Verification items for the finished model (mm, model axes). Face numbers are marked on the shaded views. A direction names the side the tool comes from. Coordinates: 2 decimals unless noted, no trailing zeros. Order: outer loops, then holes, each group sorted by start corner. A loop starts at its lowest first (then second) coordinate and runs counter-clockwise, first axis right, second up. Notation, with made-up numbers: (14, 60) -> (22, 60) arc R24 ccw to (22, 84) -> close; hole circle Ø8 at (45, 4). An arc over 180 degrees is marked (long way). Write item = value, one per line. Start each with the question number.
1. Cross-section at D-D on z = 26. Record the cut outline in (x, y), plus the area to 3 significant figures.
2. Cross-section at B-B on x = 48. Record the cut outline in (y, z).
3. Set-up check for the marked faces 1, 2, 3 and 4: record each of +Z, -Z, +X, -X, +Y, -Y from which the full face is reachable in a straight line by a thin tool's end or side.
4. Go/stop test with flat-tipped pins: P1, Ø14.5, axis at x = 32.5, y = 7, coming from the -Z side; P2, Ø2, axis at y = -3.5, z = 17.5, coming from the -X side; P3, Ø1.6, axis at y = 7, z = 19, coming from the +X side; P4, Ø2.5, axis at y = -7.5, z = -1.5, coming from the -X side. Record where each tip stops, or that it passes through.
5. Cross-section at C-C on y = 11.75. Record the cut outline in (x, z).
6. Cross-section at A-A on y = 7. Record the cut outline in (x, z).
7. Thickness scan on line 1 along Z through (x, y) = (59, 10); line 2 along Z through (x, y) = (11, -3.75); line 3 along Z through (x, y) = (45.5, -3). Record the ranges inside material, lowest first. Write a range as from..to.
8. Release check for a two-part mould opening along Z. For the marked faces 5, 6 and 7 record: +Z half, -Z half, draft (parallel to the pull), parting line (faces both ways), or undercut.
from build123d import *

# Parameters (mm, degrees)
BOSS_EXTRUDE1_DEPTH     = 94.99986
SKETCH2_W               = 23
SKETCH2_H               = 14
CUT_EXTRUDE1_DEPTH      = 2
CUT_EXTRUDE2_DEPTH      = 86.037208991
CUT_EXTRUDE2_DEPTH_BACK = 86.037208991
SKETCH4_W               = 25
SKETCH4_H               = 32.499936
SKETCH4_W_2             = 24.99986
SKETCH4_H_2             = 36
SKETCH5_W               = 25
SKETCH5_H               = 2.6
BOSS_EXTRUDE3_DEPTH     = 2
SKETCH6_W               = 24.99986
SKETCH6_H               = 2.5
BOSS_EXTRUDE4_DEPTH     = 2
SKETCH7_R               = 1.5
CUT_EXTRUDE3_DEPTH      = 10
SKETCH8_R               = 1.5
CUT_EXTRUDE4_DEPTH      = 10


with BuildPart() as part:
    # Sketch1 → Boss-Extrude1 (new body)
    with BuildSketch(Plane.ZY.offset(29.759563114)):
        Polygon((-16.355611523, -2.282836071), (-18.355611523, -2.282836071), (-18.355611523, -4.782836071), (18.644388477, -4.782836071), (18.644388477, -2.282836071), (16.644388477, -2.282836071), (16.644388477, 15.217163929), (19.644388477, 15.217163929), (19.644388477, 8.217163929), (17.644388477, 8.217163929), (17.644388477, 5.617163929), (50.644324477, 5.617163929), (50.644324477, 8.217163929), (48.644324477, 8.217163929), (48.644324477, 15.217163929), (52.144324477, 15.217163929), (52.144324477, -13.782836071), (-19.355611523, -13.782836071), (-19.355611523, -0.782836071), (-16.355611523, -0.782836071), align=None)
    extrude(amount=-BOSS_EXTRUDE1_DEPTH)

    # Sketch2 → Cut-Extrude1 (cut)
    with BuildSketch(Plane(origin=(0, 5.617163929, 0), x_dir=(1, 0, 0), z_dir=(0, 1, 0))):
        with Locations((53.740296886, -27.644388477)):
            Rectangle(SKETCH2_W, SKETCH2_H)
    extrude(amount=-CUT_EXTRUDE1_DEPTH, mode=Mode.SUBTRACT)

    # Sketch4 → Cut-Extrude2 (cut, two sides: drawn at the far end of the back side and taken through both)
    with BuildSketch(Plane(origin=(0, -0.782836071, 0), x_dir=(1, 0, 0), z_dir=(0, 1, 0)).offset(-CUT_EXTRUDE2_DEPTH_BACK)):
        with Locations((-17.259563114, -35.894356477)):
            Rectangle(SKETCH4_W, SKETCH4_H)
        with Locations((52.740366886, 1.355611523)):
            Rectangle(SKETCH4_W_2, SKETCH4_H_2)
    extrude(amount=CUT_EXTRUDE2_DEPTH + CUT_EXTRUDE2_DEPTH_BACK, mode=Mode.SUBTRACT)

    # Sketch5 → Boss-Extrude3 (add)
    with BuildSketch(Plane.XY.offset(19.644388477)):
        with Locations((-17.259563114, 6.917163929)):
            Rectangle(SKETCH5_W, SKETCH5_H)
    extrude(amount=-BOSS_EXTRUDE3_DEPTH)

    # Sketch6 → Boss-Extrude4 (add)
    with BuildSketch(Plane(origin=(0, 0, 16.644388477), x_dir=(-1, 0, 0), z_dir=(0, 0, -1))):
        with Locations((-52.740366886, -3.532836071)):
            Rectangle(SKETCH6_W, SKETCH6_H)
    extrude(amount=-BOSS_EXTRUDE4_DEPTH)

    # Sketch7 → Cut-Extrude3 (cut)
    with BuildSketch(Plane(origin=(65.240296886, 0, 0), x_dir=(0, 0, -1), z_dir=(1, 0, 0))):
        with Locations((-40.144324477, 3.217163929)):
            Circle(SKETCH7_R)
    extrude(amount=-CUT_EXTRUDE3_DEPTH, mode=Mode.SUBTRACT)

    # Sketch8 → Cut-Extrude4 (cut)
    with BuildSketch(Plane.ZY.offset(29.759563114)):
        with Locations((-1.355611523, -7.182836071)):
            Circle(SKETCH8_R)
    extrude(amount=-CUT_EXTRUDE4_DEPTH, mode=Mode.SUBTRACT)


solid = part.part
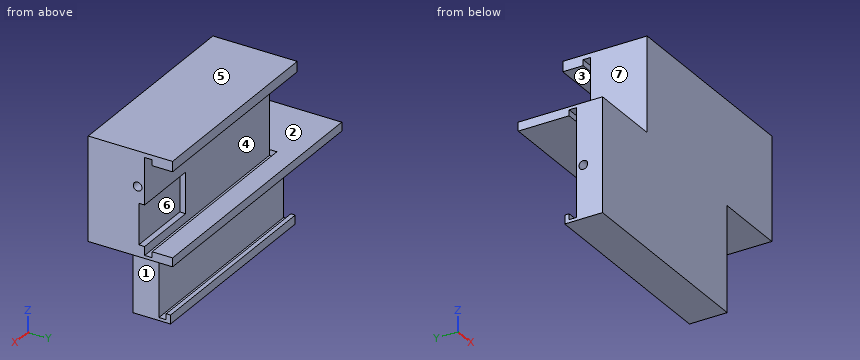
Worked out:
q1.outline = (-4.76, -13.78) -> (65.24, -13.78) -> (65.24, 3.62) -> (42.24, 3.62) -> (42.24, 5.62) -> (-4.76, 5.62) -> close
q1.area = 1,310 mm²
q2.outline = (-13.78, 16.64) -> (15.22, 16.64) -> (15.22, 19.64) -> (8.22, 19.64) -> (8.22, 17.64) -> (5.62, 17.64) -> (5.62, 20.64) -> (3.62, 20.64) -> (3.62, 34.64) -> (5.62, 34.64) -> (5.62, 50.64) -> (8.22, 50.64) -> (8.22, 48.64) -> (15.22, 48.64) -> (15.22, 52.14) -> (-13.78, 52.14) -> close
q3.face_1 = -Z, +X, +Y, -Y
q3.face_2 = -X, +Y
q3.face_3 = +X, -X, +Y
q3.face_4 = +X
q4.P1 = 16.64
q4.P2 = 40.24
q4.P3 = -4.76
q4.P4 = -29.76
q5.outline = (-29.76, 16.64) -> (65.24, 16.64) -> (65.24, 19.64) -> (-29.76, 19.64) -> close; (-4.76, 48.64) -> (65.24, 48.64) -> (65.24, 52.14) -> (-4.76, 52.14) -> close
q6.outline = (-29.76, 16.64) -> (65.24, 16.64) -> (65.24, 17.64) -> (-4.76, 17.64) -> (-4.76, 19.64) -> (-29.76, 19.64) -> close; (-4.76, 50.64) -> (65.24, 50.64) -> (65.24, 52.14) -> (-4.76, 52.14) -> close
q7.line_1 = 16.64..19.64, 48.64..52.14
q7.line_2 = -19.36..-18.36, 18.64..52.14
q7.line_3 = 16.64..52.14
q8.face_5 = +Z half
q8.face_6 = undercut
q8.face_7 = draft
